Could you check a few things on this model? Use its own coordinates, in mm. A direction names the side the tool comes from. Give positions to 0.01 mm unless a question says otherwise; leave off trailing zeros. Loops run counter-clockwise (first coordinate to the right, second up) from the corner with the lowest first, then second, coordinate; pieces in that order, holes last. Notation, with made-up numbers: (63, 54) -> (99, 54) arc R3 cw to (99, 59) -> close; hole circle Ø7 at (27, -22.5). An arc over 180 degrees is marked (long way). Write each question's results on one line, items separated by ' | '. Start each with the question number.
Q1. Will these pins go through, and if not, where does the flat tip stop? P1, Ø1.5, axis at y = -19.5, z = 1.5, coming from the -X side; P2, Ø0.9, axis at y = -19.5, z = 1, coming from the +X side; P3, Ø0.9, axis at x = 131, z = 1.5, coming from the -Y side.
Q2. We'd pull the mould along Y, two halves only. Please class faces 1 (the face through (-33, -13.573, 1)), 2 (the face through (33.638, -20, 1)), 3 (the face through (-34.362, -1, 1)): released by +Y, released by -Y, zero draft, split by the parting line, or undercut.
Q3. Which directions (+Z, -Z, +X, -X, +Y, -Y) give clear straight access to the entire face, cutting with the end or side of a thin tool? Please do faces 4 (the face through (131.638, -1, 1)), 5 (the face through (128.638, -19, 1)), 6 (the face through (-31.362, -19, 1)), 7 (the face through (53.638, -20, 1)).
Q4. If we section it at A-A, the plane x = 98: List the corners of the cut face in (y, z) for me.
Q5. If we section it at B-B, the plane z = 0.6: Give the number of separate pieces and of enclosed holes in the cut face, plus the area to 3 significant figures.
Q6. If I drill on line 1 along Y through (x, z) = (-21, 0.95); line 2 along X through (y, z) = (-15, 2.95), over which ranges is the centre line in solid material (lowest first)?
from build123d import *

# Parameters (mm, degrees)
SKETCH1_W           = 10
SKETCH1_H           = 3
BOSS_EXTRUDE1_DEPTH = 3


with BuildPart() as part:
    # Sketch1 → Boss-Extrude1 (new body)
    with BuildSketch(Plane.XY):
        Polygon((-31.361502347, 21.305164319), (128.638497653, 21.305164319), (128.638497653, 11.427031749), (131.638497653, 11.427031749), (131.638497653, -13.572968251), (128.638497653, -13.572968251), (128.638497653, -24.694835681), (-31.361502347, -24.694835681), (-31.361502347, -13.572968251), (-34.361502347, -13.572968251), (-34.361502347, 11.427031749), (-31.361502347, 11.427031749), align=None)
        with Locations((-1.361502347, -20.072968251)):
            Rectangle(SKETCH1_W, SKETCH1_H, mode=Mode.SUBTRACT)
        with Locations((-21.361502347, -20.072968251)):
            Rectangle(SKETCH1_W, SKETCH1_H, mode=Mode.SUBTRACT)
        with Locations((18.638497653, -20.072968251)):
            Rectangle(SKETCH1_W, SKETCH1_H, mode=Mode.SUBTRACT)
        with Locations((38.638497653, -20.072968251)):
            Rectangle(SKETCH1_W, SKETCH1_H, mode=Mode.SUBTRACT)
        with Locations((58.638497653, -20.072968251)):
            Rectangle(SKETCH1_W, SKETCH1_H, mode=Mode.SUBTRACT)
        with Locations((78.638497653, -20.072968251)):
            Rectangle(SKETCH1_W, SKETCH1_H, mode=Mode.SUBTRACT)
        with Locations((98.638497653, -20.072968251)):
            Rectangle(SKETCH1_W, SKETCH1_H, mode=Mode.SUBTRACT)
        with Locations((118.638497653, -20.072968251)):
            Rectangle(SKETCH1_W, SKETCH1_H, mode=Mode.SUBTRACT)
    extrude(amount=BOSS_EXTRUDE1_DEPTH)


solid = part.part
Final values:
1) P1: stops at x = -31.36 | P2: stops at x = 128.64 | P3: stops at y = -13.57
2) face 1: released by -Y | face 2: undercut | face 3: zero draft
3) face 4: +Z, -Z, +X, +Y, -Y | face 5: +Z, -Z, +X, -Y | face 6: +Z, -Z, -X, -Y | face 7: +Z, -Z
4) outline: (-24.69, 0) -> (-21.57, 0) -> (-21.57, 3) -> (-24.69, 3) -> close; (-18.57, 0) -> (21.31, 0) -> (21.31, 3) -> (-18.57, 3) -> close
5) separate pieces: 1 | enclosed holes: 8 | area: 7,270 mm²
6) line 1: y = -24.69 to -21.57, -18.57 to 21.31 | line 2: x = -31.36 to 128.64
